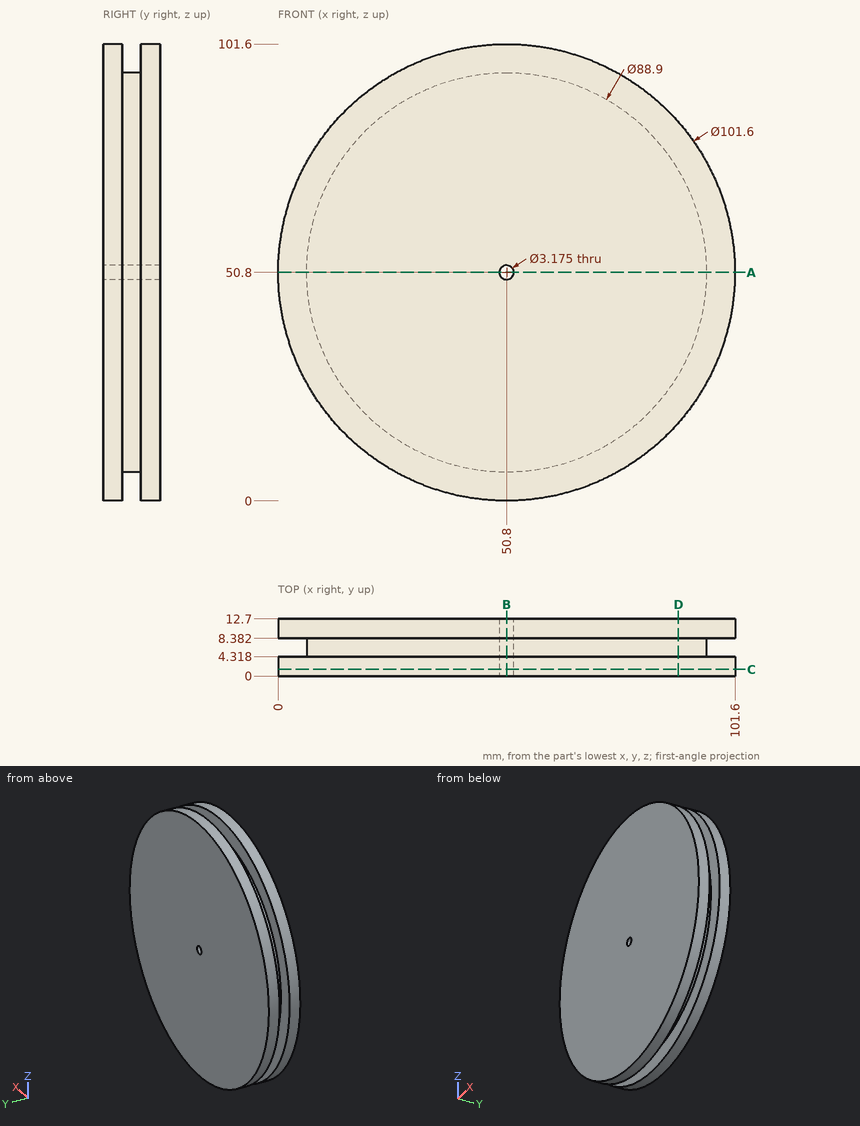
Geometry: see drawing. Coordinates: mm, zero at the bounding-box minimum. Give positions to 0.01 mm unless a question says otherwise; leave off trailing zeros. Order: outer loops, then holes, each group sorted by start corner. A loop starts at its lowest first (then second) coordinate and runs counter-clockwise, first axis right, second up. Notation, with made-up numbers: (-6.75, -34.5) - (34.25, -34.5) arc R20 cw to (34.25, -15.5) - close; hole circle Ø5 at (-15.5, -26). An arc over 180 degrees is marked (long way). Use a Markdown table: item, result.
(1) Section query D-D (x = 89). Output: boundary loops of the cut face in (y, z), then the cut area to 3 significant figures.
Computed values:
| item | result |
|---|---|
| outline | (0, 17.31) - (4.32, 17.31) - (4.32, 28.07) - (8.38, 28.07) - (8.38, 17.31) - (12.7, 17.31) - (12.7, 84.29) - (8.38, 84.29) - (8.38, 73.53) - (4.32, 73.53) - (4.32, 84.29) - (0, 84.29) - close |
| area | 763 mm2 |
(2) Section query A-A (z = 50.8). Output: boundary loops of the cut face in (x, y).
Computed values:
| item | result |
|---|---|
| outline | (0, 0) - (49.21, 0) - (49.21, 12.7) - (0, 12.7) - (0, 8.38) - (6.35, 8.38) - (6.35, 4.32) - (0, 4.32) - close; (52.39, 0) - (101.6, 0) - (101.6, 4.32) - (95.25, 4.32) - (95.25, 8.38) - (101.6, 8.38) - (101.6, 12.7) - (52.39, 12.7) - close |
(3) Section query C-C (y = 1.5). Output: boundary loops of the cut face in (x, z) (1 decimal), then the cut area to 3 significant figures.
Computed values:
| item | result |
|---|---|
| outline | circle Ø101.6 at (50.8, 50.8); hole circle Ø3.2 at (50.8, 50.8) |
| area | 8,100 mm2 |
(4) Line query: line 1 (Z direction, x = 50.5, y = 10); line 2 (Y direction, x = 32, z = 7); line 3 (Z direction, x = 49.5, y = 9). Output: solid intervals per line, ascending. Write a range as from..to.
Computed values:
| item | result |
|---|---|
| line 1 | z = 0..49.24, 52.36..101.6 |
| line 2 | y = 0..4.32, 8.38..12.7 |
| line 3 | z = 0.02..49.89, 51.71..101.58 |
(5) Pin query (flat end, axial travel): pin 1 (6 mm diameter, centred on x = 19.5, y = 2, fed in from +Z); pin 2 (5 mm diameter, centred on y = 10.5, z = 89.5, fed in from -X); pin 3 (4 mm diameter, centred on y = 9, z = 86.5, fed in from -X). Return the tip coordinate at first contact, or that it passes through.
Computed values:
| item | result |
|---|---|
| pin 1 | stops at z = 92.99 |
| pin 2 | stops at x = 15.16 |
| pin 3 | stops at x = 12.79 |
(6) Section query B-B (x = 50.8). Output: boundary loops of the cut face in (y, z), then the cut area to 3 significant figures.
Computed values:
| item | result |
|---|---|
| outline | (0, 0) - (4.32, 0) - (4.32, 6.35) - (8.38, 6.35) - (8.38, 0) - (12.7, 0) - (12.7, 49.21) - (0, 49.21) - close; (0, 52.39) - (12.7, 52.39) - (12.7, 101.6) - (8.38, 101.6) - (8.38, 95.25) - (4.32, 95.25) - (4.32, 101.6) - (0, 101.6) - close |
| area | 1,200 mm2 |
